Geometry: final body of the model. Coordinates: model frame, mm. Give positions to 0.01 mm unless a question says otherwise; leave off trailing zeros. Write each loop counter-clockwise with the first axis right and the second up, starting at its lowest first coordinate (ties: lowest second). Pieces come first, ordered by that corner, then holes. Notation, with made-up numbers: (27, 14) -> (59, 14) arc R26 cw to (59, 51) -> close; hole circle Ø8 at (64, -23). An arc over 180 degrees is marked (long way). Answer as a JSON object with one key per item and string values.
from build123d import *

# Parameters (mm, degrees)
F0_W     = 19.05
F0_H     = 25.4
F1_DEPTH = 1.016
F2_SIZE  = 2.032
F3_SIZE  = 2.032
F4_R     = 0.762
F5_R     = 0.762
F6_W     = 17.124948
F6_H     = 19.74232
F7_DEPTH = 0.1778


with BuildPart() as f1:
    # F0 (on Top) → F1 (new body)
    with BuildSketch(Plane.XY):
        with Locations((9.525, 12.7)):
            Rectangle(F0_W, F0_H)
    extrude(amount=F1_DEPTH)

    # F2
    f2_edges = [f1.edges().sort_by_distance(p)[0] for p in [
        (0, 0, 0.508),
    ]]
    chamfer(f2_edges, length=F2_SIZE)

    # F3
    f3_edges = [f1.edges().sort_by_distance(p)[0] for p in [
        (19.05, 0, 0.508),
    ]]
    chamfer(f3_edges, length=F3_SIZE)

    # F4
    f4_edges = [f1.edges().sort_by_distance(p)[0] for p in [
        (19.05, 25.4, 0.508),
    ]]
    fillet(f4_edges, radius=F4_R)

    # F5
    f5_edges = [f1.edges().sort_by_distance(p)[0] for p in [
        (0, 25.4, 0.508),
    ]]
    fillet(f5_edges, radius=F5_R)

    # F6 (on face) → F7 (cut)
    with BuildSketch(Plane.XY.offset(1.016)):
        with Locations((9.449543, 12.13214)):
            Rectangle(F6_W, F6_H)
    extrude(amount=-F7_DEPTH, mode=Mode.SUBTRACT)


solid = f1.part
Q1. First-contact query: P1, Ø5, axis at x = 14, y = 8, coming from the +Z side. Flat tip, straight axial feed; report the tip coordinate or a pass-through.
Values:
{"P1": "z = 0.84"}
Q2. Mould query, pull axis Y, two halves, no side actions, for faces 1 (the flat face through (9.4, 0, 0.5)), 2 (the flat face through (9, 12, 0.838)), 3 (the flat face through (9.4, 25.4, 0.5)), 4 (the flat face through (8.8, 22.2, 1.016)). Classes: pulls with the +Y half, pulls with the -Y half, needs draft (parallel to the pull), parting line crosses it, or undercut.
Values:
{"face 1": "pulls with the -Y half", "face 2": "undercut", "face 3": "pulls with the +Y half", "face 4": "needs draft"}
Q3. Material intervals for L1, parallel to Y at x = 8.75, z = 0.9; L2, parallel to X at y = 12.5, z = 0.95; L3, parallel to Z at x = 3.5, y = 20.25, sorted ascending. Write a range as from..to.
Values:
{"L1": "0..2.26, 22..25.4", "L2": "0..0.89, 18.01..19.05", "L3": "0..0.84"}
Q4. Cut plane A-A (y = 8). Return the cut outline in (x, z), and give its area (3 significant figures).
Values:
{"outline": "(0, 0) -> (19.05, 0) -> (19.05, 1.02) -> (18.01, 1.02) -> (18.01, 0.84) -> (0.89, 0.84) -> (0.89, 1.02) -> (0, 1.02) -> close", "area": "16.3 mm²"}
Q5. Cut plane B-B (x = 14). Return the cut outline in (y, z).
Values:
{"outline": "(0, 0) -> (25.4, 0) -> (25.4, 1.02) -> (22, 1.02) -> (22, 0.84) -> (2.26, 0.84) -> (2.26, 1.02) -> (0, 1.02) -> close"}
